Check sheet for the drawn part. Datum: minimum x, y, z corner. Units: mm. A direction names the side the tool comes from. Give positions to 0.01 mm unless a question says otherwise; leave off trailing zeros. Order: outer loops, then holes, each group sorted by start corner. A loop starts at its lowest first (then second) coordinate and runs counter-clockwise, first axis right, second up. Notation, with made-up numbers: M -18,-32 L -5,-32 A23 cw -5,-14 Z; hole C 26.25,71 d10. An arc over 180 degrees is marked long. Answer in a Markdown table with one row per item. Add a question column.
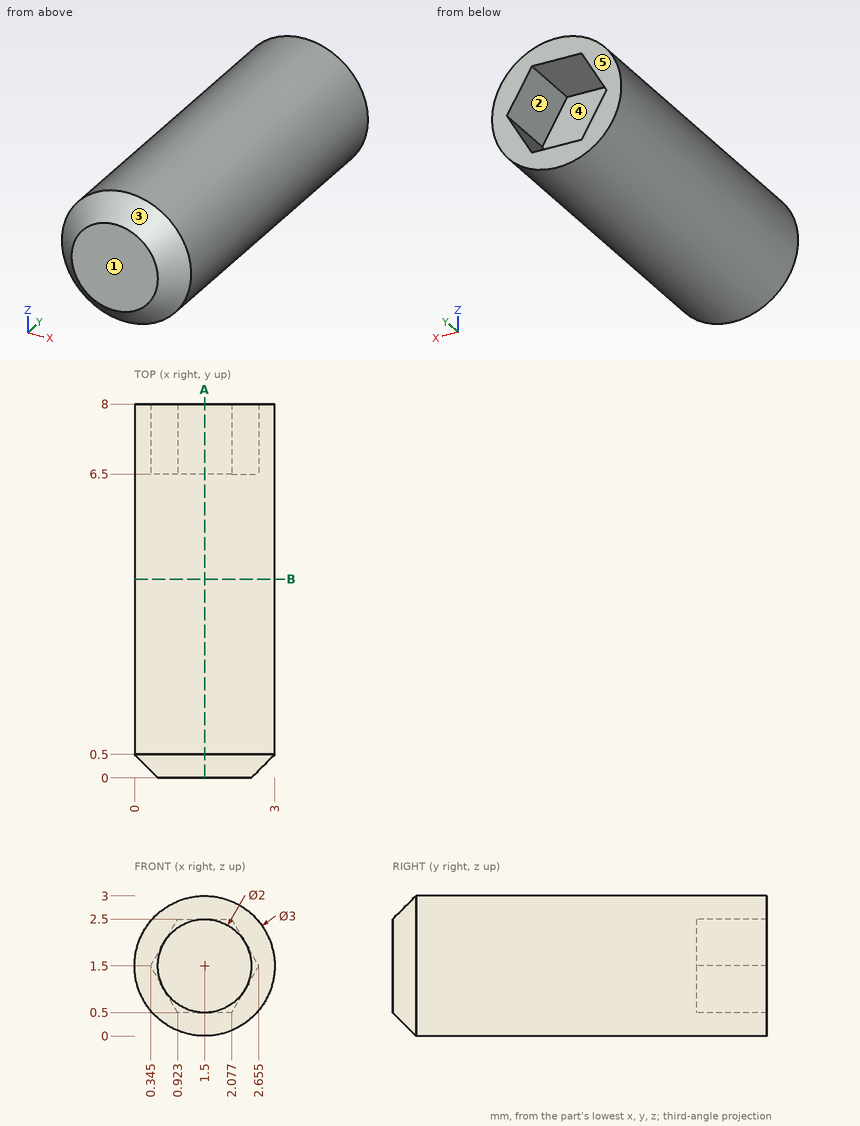
Q1. Tool access check on the marked faces 4 and 5. Record the directions out of +Z, -Z, +X, -X, +Y, -Y that give a thin tool (end or side, any length) a straight path to the whole face; none if there is none.
Q2. Go/stop test with a flat-tipped pin: pin 1 (1 mm diameter, centred on x = 1.5, z = 1.5, fed in from +Y). Record where the tip stops, or that it passes through.
Q3. Thickness scan on probe 1 along X at (y, z) = (6.75, 1.55) (1 decimal); probe 2 along X at (y, z) = (7.25, 0.85); probe 3 along Y at (x, z) = (1.45, 0.8). Record the ranges inside material, lowest first.
Q4. Draft check along X on the marked faces 1, 2 and 3. Enter one of: pulls with the +X half, pulls with the -X half, needs draft (parallel to the pull), parting line crosses it, or undercut.
Q5. Cross-section at A-A (x = 1.5). Record the boundary of the cut face in (y, z).
Q6. Cross-section at B-B (y = 4.25). Record the boundary of the cut face in (x, z).
Values follow:
| question | item | result |
|---|---|---|
| 1 | face 4 | +Y |
| 1 | face 5 | +Z, -Z, +X, -X, +Y |
| 2 | pin 1 | y = 6.5 |
| 3 | probe 1 | 0 to 0.4, 2.6 to 3 |
| 3 | probe 2 | 0.15 to 0.72, 2.28 to 2.85 |
| 3 | probe 3 | 0 to 6.5 |
| 4 | face 1 | needs draft |
| 4 | face 2 | undercut |
| 4 | face 3 | parting line crosses it |
| 5 | outline | M 0,0.5 L 0.5,0 L 8,0 L 8,0.5 L 6.5,0.5 L 6.5,2.5 L 8,2.5 L 8,3 L 0.5,3 L 0,2.5 Z |
| 6 | outline | C 1.5,1.5 d3 |
